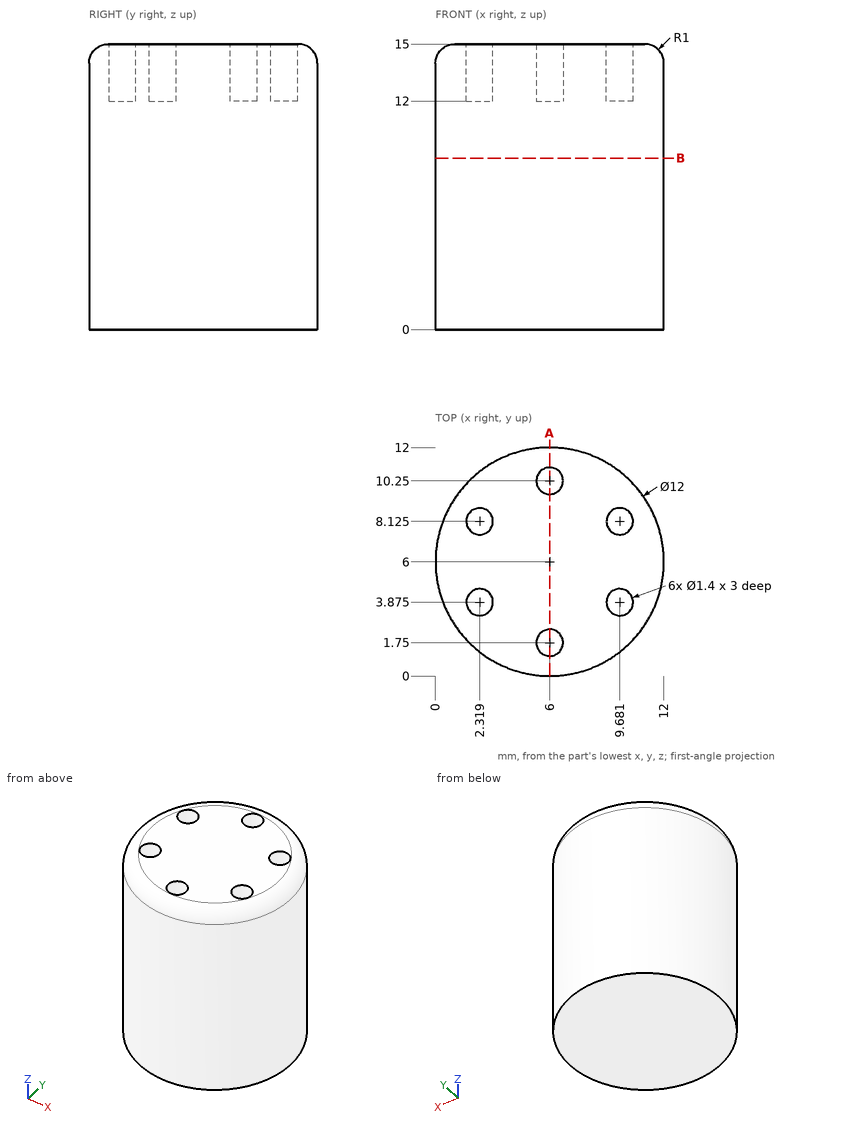
Input: dimensioned drawing with shaded views. Units: mm. Origin: part minimum x, y, z. Coordinates: 2 decimals unless noted, no trailing zeros. Loops run counter-clockwise (first coordinate to the right, second up) from the corner with the lowest first, then second, coordinate; pieces in that order, holes last.
Q1. Contact query for flat-ended pins moving along their axis: pin 1 (1.5 mm diameter, centred on x = 10.5, y = 2, fed in from +Z); pin 2 (1.1 mm diameter, centred on x = 6, y = 1.75, fed in from +Z); pin 3 (1.5 mm diameter, centred on y = 7, z = 3.5, fed in from -X) (1 decimal). Output: stop coordinate, or through.
Results are:
pin 1: stops at z = 14.96
pin 2: stops at z = 12
pin 3: stops at x = 0
Q2. Section A-A, the plane x = 6. Return the cut outline in (y, z).
Results are:
outline: (0, 0) - (12, 0) - (12, 14) arc R1 ccw to (11, 15) - (10.95, 15) - (10.95, 12) - (9.55, 12) - (9.55, 15) - (2.45, 15) - (2.45, 12) - (1.05, 12) - (1.05, 15) - (1, 15) arc R1 ccw to (0, 14) - close
Q3. Section B-B, the plane z = 9. Return the cut outline in (x, y).
Results are:
outline: circle Ø12 at (6, 6)
Q4. Line query: line 1 along Y through (x, z) = (6, 13.9); line 2 along Y through (x, z) = (6, 14.35); line 3 along X through (y, z) = (1.75, 12.25) (1 decimal). Output: solid intervals per line, ascending.
Results are:
line 1: y = 0 to 1.05, 2.45 to 9.55, 10.95 to 12
line 2: y = 0.06 to 1.05, 2.45 to 9.55, 10.95 to 11.94
line 3: x = 1.8 to 5.3, 6.7 to 10.2
